Check sheet for the modelled part. Datum: model origin and axes. Units: mm. Round coordinates to 2 decimals unless told otherwise and drop trailing zeros. Write each loop counter-clockwise with the first axis right and the second up, starting at its lowest first coordinate (ties: lowest second). Pieces come first, ordered by that corner, then holes. Notation, with made-up numbers: M -14,56.5 L 11,56.5 A33 ccw 11,84.5 Z; hole C -14,-38.5 d7. An arc over 180 degrees is marked long. One line per item, written item: value.
Autodesk Inventor part; units mm, degrees
ref_plane "YZ Plane" through (0, 0, 0) normal (1, 0, 0) x (0, 1, 0)
ref_plane "XZ Plane" through (0, 0, 0) normal (0, 1, 0) x (-1, 0, 0)
ref_plane "XY Plane" through (0, 0, 0) normal (0, 0, 1) x (1, 0, 0)
sketch "Sketch1" plane through (0, 0, 0) normal (0, 0, 1) x (1, 0, 0)
  line L0 (73.66, -76.2) -> (-84.709, -76.2)
  line L1 (-84.709, -76.2) -> (-84.709, 50.8)
  line L2 (-84.709, 50.8) -> (73.66, 50.8)
  line L3 (73.66, 50.8) -> (73.66, -76.2)
  line L4 (-84.709, 50.8) -> (-32, 50.8)
  line L5 (-32, 50.8) -> (-32, 38.1)
  line L6 (-32, 38.1) -> (-84.709, 38.1)
  line L7 (-84.709, 38.1) -> (-84.709, 50.8)
  line L8 (73.66, 50.8) -> (32, 50.8)
  line L9 (32, 50.8) -> (32, -22.225)
  line L10 (32, -22.225) -> (73.66, -22.225)
  line L11 (73.66, -22.225) -> (73.66, 50.8)
  line L12 (-34.4202, -12.5158) -> (-52.8352, -12.5158)
  line L13 (-52.8352, -12.5158) -> (-52.8352, -5.5308)
  line L14 (-52.8352, -5.5308) -> (-34.4202, -5.5308)
  line L15 (-34.4202, -5.5308) -> (-34.4202, -12.5158)
  line L16 (-34.4202, -12.5158) -> (-52.8352, -5.5308) construction
  line L17 (-52.8352, -12.5158) -> (-34.4202, -5.5308) construction
  line L18 (-34.4202, -63.3158) -> (-52.8352, -63.3158)
  line L19 (-52.8352, -63.3158) -> (-52.8352, -56.3308)
  line L20 (-52.8352, -56.3308) -> (-34.4202, -56.3308)
  line L21 (-34.4202, -56.3308) -> (-34.4202, -63.3158)
  line L22 (-34.4202, -63.3158) -> (-52.8352, -56.3308) construction
  line L23 (-52.8352, -63.3158) -> (-34.4202, -56.3308) construction
  line L24 (48.7648, -63.3158) -> (67.1798, -63.3158)
  line L25 (67.1798, -63.3158) -> (67.1798, -56.3308)
  line L26 (67.1798, -56.3308) -> (48.7648, -56.3308)
  line L27 (48.7648, -56.3308) -> (48.7648, -63.3158)
  line L28 (48.7648, -63.3158) -> (67.1798, -56.3308) construction
  line L29 (67.1798, -63.3158) -> (48.7648, -56.3308) construction
  line L30 (-43.6277, -59.8233) -> (-43.6277, -9.0233) construction
  line L31 (-43.6277, -59.8233) -> (-43.6277, -56.3308) construction
  line L32 (-25, 43.8) -> (25, 43.8) construction
  line L33 (25, 43.8) -> (25, -6.2) construction
  line L34 (25, -6.2) -> (-25, -6.2) construction
  line L35 (-25, -6.2) -> (-25, 43.8) construction
  line L36 (-25, 18.8) -> (25, 18.8) construction
  line L37 (57.9723, -59.8233) -> (-43.6277, -59.8233) construction
  line L38 (0, 43.8) -> (0, -6.2) construction
  line L39 (32, -13.2) -> (-32, -13.2) construction
  line L40 (-32, -13.2) -> (-32, 50.8) construction
  line L41 (-32, 50.8) -> (32, 50.8) construction
  line L42 (32, 50.8) -> (32, -13.2) construction
  line L43 (32, -13.2) -> (-32, 50.8) construction
  line L44 (-32, -13.2) -> (32, 50.8) construction
  circle A0 centre (-37.6333, -9.0233) radius 3.0299 construction
  circle A1 centre (-43.6277, -9.0233) radius 2.9972 construction
  circle A2 centre (-37.6333, -9.0233) radius 4.7625 construction
  line L45 (0, 76.2) -> (0, -101.6)
  line L46 (57.9723, -59.8233) -> (57.9723, -34.4233) construction
  line L47 (67.1798, -30.9308) -> (48.7648, -30.9308)
  line L48 (48.7648, -30.9308) -> (48.7648, -37.9158)
  line L49 (48.7648, -37.9158) -> (67.1798, -37.9158)
  line L50 (67.1798, -37.9158) -> (67.1798, -30.9308)
  line L51 (67.1798, -30.9308) -> (48.7648, -37.9158) construction
  line L52 (48.7648, -30.9308) -> (67.1798, -37.9158) construction
  point P0 (0, 0)
  point P1 (0, 0)
  point P2 (0, 0)
  point P3 (0, 18.8)
  dimension "d1" = 127
  dimension "d2" = 12.7
  dimension "d24" = 6.985
  dimension "d25" = 18.415
  dimension "d26" = 6.985
  dimension "d34" = 6.985
  dimension "d40" = 50
  dimension "d41" = 50
  dimension "d45" = 101.6
  dimension "d48" = 59.8233
  dimension "d49" = 50.8
  dimension "d50" = 64
  dimension "d51" = 64
  dimension "d52" = 0
  dimension "d53" = 5.9944
  dimension "d54" = 5.9944
  dimension "d57" = 50.8
  dimension "d60" = 9.525
  dimension "d61" = 73.025
  dimension "d63" = 64
  dimension "d64" = 0
  dimension "d65" = 84.709
  dimension "d66" = 73.66
  dimension "d67" = 43.6277
  dimension "d68" = 6.4802
  dimension "d69" = 158.369
  dimension "d70" = 31.8738
  dimension "d71" = 25.4
extrude "Extrusion1" add sketch "Sketch1" along normal blind 9.525 contours L0 L45 L2 L9 L10 L3 | L0 L1 L6 L5 L2 L45 | L12 L13 L14 L15 | L18 L19 L20 L21 | L27 L26 L25 L24 | L50 L49 L48 L47
hole "Hole1" at (-25, 43.8, 0) at (25, 43.8, 0) at (25, -6.2, 0) at (-25, -6.2, 0) direction (0, 0, 1) diameter 4.9276 end through all
extrude "Extrusion2" cut sketch "Sketch1" along normal up to next contours L12 L13 L14 L15 | L18 L19 L20 L21 | L27 L26 L25 L24 | L50 L49 L48 L47
sketch "Sketch3" plane through (0, 0, 9.525) normal (0, 0, 1) x (1, 0, 0)
  line L0 (73.66, -22.225) -> (32, -22.225)
  line L1 (32, -22.225) -> (32, 50.8)
  line L2 (27.6058, -24.9428) -> (50.6944, -24.9428)
  line L3 (50.6944, -24.9428) -> (50.6944, -9.9084)
  line L4 (50.6944, -9.9084) -> (27.6058, -9.9084)
  line L5 (27.6058, -9.9084) -> (27.6058, -24.9428)
  point P0 (0, 0)
  dimension "d99" = 23.0886
  dimension "d100" = 2.7178
  dimension "d101" = 4.3942
extrude "Extrusion4" cut sketch "Sketch3" against normal blind 6.731
fillet "Fillet1" radius 3.175 8 edges at (-32, 38.1, 4.7625) (-32, 50.8, 4.7625) (32, 50.8, 4.7625) (73.66, -22.225, 4.7625) (-84.709, 38.1, 4.7625) (-84.709, -76.2, 4.7625) (73.66, -76.2, 4.7625) (32, -22.225, 1.397)
fillet "Fillet2" radius 3.175 16 edges at (-52.8352, -63.3158, 4.7625) (-52.8352, -12.5158, 4.7625) (-52.8352, -56.3308, 4.7625) (-52.8352, -5.5308, 4.7625) (48.7648, -63.3158, 4.7625) (48.7648, -56.3308, 4.7625) (67.1798, -56.3308, 4.7625) (67.1798, -63.3158, 4.7625) (-34.4202, -5.5308, 4.7625) (-34.4202, -12.5158, 4.7625) (-34.4202, -56.3308, 4.7625) (-34.4202, -63.3158, 4.7625) (48.7648, -30.9308, 4.7625) (48.7648, -37.9158, 4.7625) (67.1798, -30.9308, 4.7625) (67.1798, -37.9158, 4.7625)
sketch "Sketch2" plane through (0, 0, 0) normal (0, 0, 1) x (1, 0, 0)
  line L0 (-72.009, 18.796) -> (-46.609, 18.796) construction
  line L1 (-46.609, 18.796) -> (-46.609, -32.004) construction
  line L2 (-46.609, -32.004) -> (-72.009, -32.004) construction
  line L3 (-72.009, -32.004) -> (-72.009, 18.796) construction
  line L4 (-35.175, 38.1) -> (-81.534, 38.1) construction
  line L5 (-84.709, 34.925) -> (-84.709, -73.025) construction
  line L6 (-52.8352, -9.3408) -> (-52.8352, -8.7058) construction
  line L7 (-52.8352, -9.0233) -> (-63.8216, -9.0233) construction
  point P0 (0, 0)
  dimension "d73" = 25.4
  dimension "d74" = 50.8
  dimension "d75" = 19.304
  dimension "d76" = 12.7
  dimension "d77" = 47.1232
hole "Hole2" at (-72.009, 18.796, 0) at (-46.609, 18.796, 0) at (-46.609, -32.004, 0) at (-72.009, -32.004, 0) direction (0, 0, 1) diameter 4.1402 end through all
fillet "Fillet5" radius 1.651 4 edges at (32, -9.9084, 6.1595) (27.6058, -9.9084, 6.1595) (27.6058, -24.9428, 6.1595) (50.6944, -24.9428, 6.1595)
sketch "Sketch4" plane through (0, 0, 9.525) normal (0, 0, 1) x (1, 0, 0)
  line L0 (57.9723, -34.4233) -> (57.9723, -59.8233) construction
  line L1 (57.9723, -47.1233) -> (65.2526, -47.1233) construction
  line L2 (73.66, -73.025) -> (73.66, -25.4) construction
  point P0 (0, 0)
  point P1 (3.6576, -47.1233)
  point P2 (3.6576, -30.6133)
  dimension "d107" = 8.4074
  dimension "d115" = 61.595
  dimension "d116" = 16.51
hole "Hole3" at (65.2526, -47.1233, 9.525) at (3.6576, -47.1233, 9.525) at (3.6576, -30.6133, 9.525) direction (0, 0, -1) diameter 4.1402 end through all
properties part number "J005167" material "ALUMINUM, 6061-T651"
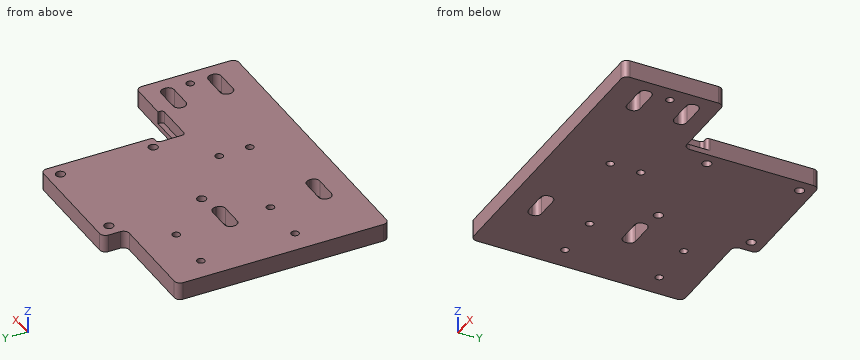
Q1. Depth check by flat-ended pin: P1, Ø10, axis at x = 41, y = -5.5, coming from the -Z side; P2, Ø1, axis at y = 1.5, z = 3, coming from the +X side; P3, Ø4, axis at x = -37.5, z = 6.5, coming from the +Y side. Enter the tip coordinate at first touch or a pass-through.
Completed:
P1: through
P2: x = 32
P3: y = 38.1
Q2. Scan lines: line 1 (Y direction, x = -25, z = 4.75); line 2 (X direction, y = 43.8, z = 4.75); line 3 (Y direction, x = 29.5, z = 7.25). Record each from-to range of solid material in increasing order. Write a range as [from, to].
Completed:
line 1: [-76.2, -8.66], [-3.74, 41.34], [46.26, 50.8]
line 2: [-32, -27.46], [-22.54, 22.54], [27.46, 32]
line 3: [-76.2, -24.94], [-9.91, 50.73]
Q3. Sectioned sample at A-A on y = 43.8. Enter the section's corners in (x, z) (3 decimals).
Completed:
outline: M -32,0 L -27.464,0 L -27.464,9.525 L -32,9.525 Z; M -22.536,0 L 22.536,0 L 22.536,9.525 L -22.536,9.525 Z; M 27.464,0 L 32,0 L 32,9.525 L 27.464,9.525 Z
Q4. Sectioned sample at B-B on x = 25. Enter the section's corners in (y, z) (3 decimals), and give its area (3 significant figures).
Completed:
outline: M -76.2,0 L -8.664,0 L -8.664,9.525 L -76.2,9.525 Z; M -3.736,0 L 41.336,0 L 41.336,9.525 L -3.736,9.525 Z; M 46.264,0 L 50.8,0 L 50.8,9.525 L 46.264,9.525 Z
area: 1,120 mm^2
